Autodesk Inventor part; units mm, degrees
ref_plane "YZ Plane" through (0, 0, 0) normal (1, 0, 0) x (0, 1, 0)
ref_plane "XZ Plane" through (0, 0, 0) normal (0, 1, 0) x (-1, 0, 0)
ref_plane "XY Plane" through (0, 0, 0) normal (0, 0, 1) x (1, 0, 0)
sketch "Sketch1" plane through (0, 0, 0) normal (0, 0, 1) x (1, 0, 0)
  line L0 (-100, -50) -> (100, -50)
  line L1 (100, -50) -> (100, 50)
  line L2 (100, 50) -> (-100, 50)
  line L3 (-100, 50) -> (-100, -50)
  line L4 (-100, -50) -> (100, 50) construction
  line L5 (100, -50) -> (-100, 50) construction
  line L6 (-63, -23) -> (63, -23)
  line L7 (63, -23) -> (63, 23)
  line L8 (63, 23) -> (-63, 23)
  line L9 (-63, 23) -> (-63, -23)
  line L10 (-63, -23) -> (63, 23) construction
  line L11 (63, -23) -> (-63, 23) construction
  point P0 (0, 0)
  dimension "d0" = 200
  dimension "d1" = 100
  dimension "d2" = 126
  dimension "d3" = 46
extrude "Extrusion1" add sketch "Sketch1" along normal blind 6
sketch "Sketch2" plane through (0, 0, 6) normal (0, 0, 1) x (1, 0, 0)
  line L0 (-80, -15) -> (80, -15)
  line L1 (80, -15) -> (80, 15)
  line L2 (80, 15) -> (-80, 15)
  line L3 (-80, 15) -> (-80, -15)
  line L4 (-80, -15) -> (80, 15) construction
  line L5 (80, -15) -> (-80, 15) construction
  point P0 (0, 0)
  dimension "d6" = 160
  dimension "d7" = 30
extrude "Extrusion2" cut sketch "Sketch2" against normal through all
sketch "Sketch3" plane through (0, 0, 6) normal (0, 0, 1) x (1, 0, 0)
  line L0 (-90.4385, 41.5009) -> (-72.2585, 41.5009) construction
  line L1 (-72.2585, 41.5009) -> (-72.2585, 36.1823) construction
  line L2 (-72.2585, 36.1823) -> (-90.4385, 36.1823) construction
  line L3 (-90.4385, 36.1823) -> (-90.4385, 41.5009) construction
  circle A0 centre (-80, 23) radius 0.25
  line L4 (-80, -15) -> (-80, 15)
  line L5 (-63, 23) -> (63, 23)
  line L6 (100, -50) -> (100, 50)
  line L7 (100, 50) -> (-100, 50)
  line L8 (-100, 50) -> (-100, -50)
  line L9 (-100, -50) -> (100, -50)
  line L10 (63, 15) -> (80, 15)
  line L11 (80, 15) -> (80, -15)
  line L12 (80, -15) -> (63, -15)
  line L13 (63, -15) -> (63, -23)
  line L14 (63, -23) -> (-63, -23)
  line L15 (-63, -23) -> (-63, -15)
  line L16 (-63, -15) -> (-80, -15)
  line L17 (-80, -15) -> (-80, 15)
  line L18 (-80, 15) -> (-63, 15)
  line L19 (-63, 15) -> (-63, 23)
  line L20 (-63, 23) -> (63, 23)
  line L21 (63, 23) -> (63, 15)
  point P0 (0, 0)
  dimension "d10" = 0
  dimension "d11" = 0
  dimension "d12" = 0.5
extrude "Extrusion3" cut sketch "Sketch3" against normal through all contours A0
properties part number "EngravingJig"
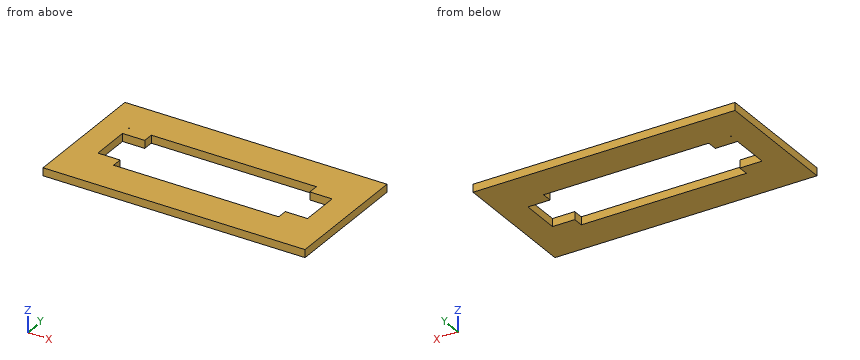
Model file for the job. Use its own axes, mm. Give positions to 0.01 mm unless a question says otherwise; leave off trailing zeros. Loops run counter-clockwise (first coordinate to the right, second up) from the corner with the lowest first, then second, coordinate; pieces in that order, holes last. Notation, with made-up numbers: (21, -2) -> (63, -2) arc R17 cw to (63, 9) -> close; hole circle Ø3 at (22, -39.5). An arc over 180 degrees is marked (long way). Use CSV: the item, a comma, the result in double quotes. Start each with the question number.
1) Wall check: line 1 (Y direction, x = 45.5, z = 3.95); line 2 (X direction, y = 2, z = 5.6). Give the ranges that are in metal, low to high.
2) Slice it at B-B on y = -19. Give the cut face in (x, z), plus the area to 3 significant figures.
3) Slice it at A-A on x = 70. Give the cut face in (y, z).
4) Flat gauge pin, fed straight in: pin 1 Ø10 at (x, y) = (18, 29) entering from -Z. Where does the tip first touch, or does it go through?
5) Slice it at C-C on z = 4.8. Give the cut face in (x, y), plus the area to 3 significant figures.
Computed values:
1,line 1,"y = -50 to -23, 23 to 50"
1,line 2,"x = -100 to -80, 80 to 100"
2,outline,"(-100, 0) -> (-63, 0) -> (-63, 6) -> (-100, 6) -> close; (63, 0) -> (100, 0) -> (100, 6) -> (63, 6) -> close"
2,area,"444 mm^2"
3,outline,"(-50, 0) -> (-15, 0) -> (-15, 6) -> (-50, 6) -> close; (15, 0) -> (50, 0) -> (50, 6) -> (15, 6) -> close"
4,pin 1,"stops at z = 0"
5,outline,"(-100, -50) -> (100, -50) -> (100, 50) -> (-100, 50) -> close; hole circle Ø0.5 at (-80, 23); hole (-80, -15) -> (-63, -15) -> (-63, -23) -> (63, -23) -> (63, -15) -> (80, -15) -> (80, 15) -> (63, 15) -> (63, 23) -> (-63, 23) -> (-63, 15) -> (-80, 15) -> close"
5,area,"13,200 mm^2"
